from build123d import *

# Parameters (mm, degrees)
SKETCH_2_W          = 1.2
SKETCH_2_H          = 2.7
EXTRUDE_1_DEPTH     = 2.5
SKETCH_3_W          = 12
SKETCH_3_H          = 2.7
EXTRUDE_2_DEPTH     = 1.2
CUT_EXTRUDE_1_DEPTH = 8


with BuildPart() as part:
    # Sketch 1 → Revolve 1 (revolve)
    with BuildSketch(Plane(origin=(0, 0, 0), x_dir=(0, 0, -1), z_dir=(1, 0, 0))):
        Polygon((-20.5, 0), (-20.5, 12), (-1.5, 12), (-1.5, 10), (0, 10), (0, 4), (6.5, 4), (6.5, 3), (16.5, 3), (16.5, 0), align=None)
    revolve(axis=Axis((0, 0, 20.5), (0, 0, -1)))



with BuildPart() as body_2:
    # Sketch 2 → Extrude 1 (new body)
    with BuildSketch(Plane(origin=(0, 0, 0), x_dir=(-1, 0, 0), z_dir=(0, 0, -1))):
        with Locations((-11.4, 0)):
            Rectangle(SKETCH_2_W, SKETCH_2_H)
    extrude(amount=EXTRUDE_1_DEPTH)


with BuildPart() as part_1:
    add(part.part)

    add(body_2.part)  # Extrude 2 merges body 2
    # Sketch 3 → Extrude 2 (add)
    with BuildSketch(Plane.XY):
        with Locations((6, 0)):
            Rectangle(SKETCH_3_W, SKETCH_3_H)
    extrude(amount=EXTRUDE_2_DEPTH)

    # Sketch 4 → Cut-Extrude 1 (cut)
    with BuildSketch(Plane(origin=(0, 0, -16.5), x_dir=(-1, 0, 0), z_dir=(0, 0, -1))):
        with BuildLine():
            Line((-1.5, 2.598076211), (-1.5, -2.598076211))
            ThreePointArc((-1.5, -2.598076211), (-3, 0), (-1.5, 2.598076211))
        make_face()
    extrude(amount=-CUT_EXTRUDE_1_DEPTH, mode=Mode.SUBTRACT)


solid = part_1.part
Input: part model. Units: mm. Frame: model coordinates. A direction names the side the tool comes from. Give positions to 0.01 mm unless a question says otherwise; leave off trailing zeros. Order: outer loops, then holes, each group sorted by start corner. A loop starts at its lowest first (then second) coordinate and runs counter-clockwise, first axis right, second up.
Q1. Section C-C on z = 12.5. Output: boundary loops of the cut face in (x, y), and give its area (3 significant figures).
Checked values:
outline: circle Ø24 at (0, 0)
area: 452 mm2
Q2. Section D-D on y = 7. Output: boundary loops of the cut face in (x, z).
Checked values:
outline: (-9.75, 1.5) - (-7.14, 1.5) - (-7.14, 0) - (7.14, 0) - (7.14, 1.5) - (9.75, 1.5) - (9.75, 20.5) - (-9.75, 20.5) - close
Q3. Section B-B on y = 0. Output: boundary loops of the cut face in (x, z), and give its area (3 significant figures).
Checked values:
outline: (-12, 1.5) - (-10, 1.5) - (-10, 0) - (-4, 0) - (-4, -6.5) - (-3, -6.5) - (-3, -16.5) - (1.5, -16.5) - (1.5, -8.5) - (3, -8.5) - (3, -6.5) - (4, -6.5) - (4, 0) - (10.8, 0) - (10.8, -2.5) - (12, -2.5) - (12, 1.2) - (10, 1.2) - (10, 1.5) - (12, 1.5) - (12, 20.5) - (-12, 20.5) - close
area: 591 mm2
Q4. Ray query, probe 1 along Z at (x, y) = (3.75, 2.5); probe 2 along Z at (x, y) = (10.75, 4.5); probe 3 along X at (y, z) = (-0.25, 6.5). Return the intervals inside material, ascending.
Checked values:
probe 1: z = 0 to 20.5
probe 2: z = 1.5 to 20.5
probe 3: x = -12 to 12
Q5. Set-up query: faces 1 (the flat face through (1.5, 0, -13)), 2 (the flat face through (-4, 2, 0)), 3 (the flat face through (11, 1.35, 0)). Return all of +Z, -Z, +X, -X, +Y, -Y with unobstructed straight access to the full face (end or side cutting, diameter ignored); none if empty.
Checked values:
face 1: -Z, +X, +Y, -Y
face 2: -Z
face 3: -Z, +X, +Y
Q6. Draft query along X for faces 4 (the flat face through (10.8, 0, -1)), 5 (the cylindrical face through (-9.76, -2.17, 0.74)), 6 (the flat face through (9, -5, 1.5)). Return one class per face: +X half, -X half, draft (parallel to the pull), parting line (faces both ways), or undercut.
Checked values:
face 4: undercut
face 5: parting line
face 6: draft
Q7. Contact query for flat-ended pins moving along their axis: pin 1 Ø1 at (x, z) = (-7.5, 13.5) entering from +Y; pin 2 Ø2.5 at (x, z) = (11, -1) entering from -Y; pin 3 Ø1.2 at (x, y) = (2.5, 0) entering from -Z. Output: stop coordinate, or through.
Checked values:
pin 1: stops at y = 9.75
pin 2: stops at y = -1.35
pin 3: stops at z = -8.5
Q8. Section A-A on x = 0. Output: boundary loops of the cut face in (y, z).
Checked values:
outline: (-12, 1.5) - (-10, 1.5) - (-10, 0) - (-4, 0) - (-4, -6.5) - (-3, -6.5) - (-3, -16.5) - (3, -16.5) - (3, -6.5) - (4, -6.5) - (4, 0) - (10, 0) - (10, 1.5) - (12, 1.5) - (12, 20.5) - (-12, 20.5) - close
